The listing builds one solid part. Answer for the finished solid, in the listing's coordinates (mm). Face numbers are marked on the shaded views. A direction names the side the tool comes from. Give positions to 0.01 mm unless a question says otherwise; leave off trailing zeros. Order: outer loops, then holes, each group sorted by start corner. A loop starts at its lowest first (then second) coordinate and runs counter-clockwise, first axis right, second up.
```python
from build123d import *

# Parameters (mm, degrees)
SKETCH1_W           = 18
SKETCH1_H           = 30
BOSS_EXTRUDE1_DEPTH = 5
SKETCH2_W           = 30
SKETCH2_H           = 30
BOSS_EXTRUDE2_DEPTH = 5
SKETCH3_R           = 1.2
CUT_EXTRUDE1_DEPTH  = 5
FILLET1_R           = 6
BOSS_EXTRUDE3_START = 4
SKETCH4_R           = 3
SKETCH4_R_2         = 1.2
BOSS_EXTRUDE3_DEPTH = 4
SKETCH5_R           = 1.7
CUT_EXTRUDE2_DEPTH  = 24
SKETCH6_R           = 3
CUT_EXTRUDE3_DEPTH  = 24
FILLET2_R           = 3


with BuildPart() as part:
    # Sketch1 → Boss-Extrude1 (new body)
    with BuildSketch(Plane(origin=(0, 0, 0), x_dir=(1, 0, 0), z_dir=(0, 1, 0))):
        with Locations((9, 15)):
            Rectangle(SKETCH1_W, SKETCH1_H)
    extrude(amount=BOSS_EXTRUDE1_DEPTH)

    # Sketch2 → Boss-Extrude2 (add)
    with BuildSketch(Plane(origin=(18, 0, 0), x_dir=(0, 0, -1), z_dir=(1, 0, 0))):
        with Locations((15, 15)):
            Rectangle(SKETCH2_W, SKETCH2_H)
    extrude(amount=-BOSS_EXTRUDE2_DEPTH)

    # Sketch3 → Cut-Extrude1 (cut)
    with BuildSketch(Plane(origin=(18, 0, 0), x_dir=(0, 0, -1), z_dir=(1, 0, 0))):
        with Locations((4.25, 27)):
            Circle(SKETCH3_R)
        with Locations((25.75, 27)):
            Circle(SKETCH3_R)
        with Locations(Location((25.75, 14.5, 0), (0, 0, 180))):
            Circle(SKETCH3_R)
        with Locations(Location((4.25, 14.5, 0), (0, 0, 180))):
            Circle(SKETCH3_R)
    extrude(amount=-CUT_EXTRUDE1_DEPTH, mode=Mode.SUBTRACT)

    # Fillet1
    fillet1_edges = [part.edges().sort_by_distance(p)[0] for p in [
        (13, 5, -15),
        (18, 0, -15),
    ]]
    fillet(fillet1_edges, radius=FILLET1_R)

    # Sketch4 → Boss-Extrude3 (add)
    # profile 1 of 4: a face of its own
    with BuildSketch(Plane(origin=(18, 0, 0), x_dir=(0, 0, -1), z_dir=(1, 0, 0)).offset(BOSS_EXTRUDE3_START)):
        with Locations(Location((4.25, 27, 0), (0, 0, 90))):
            Circle(SKETCH4_R)
        with Locations((4.25, 27)):
            Circle(SKETCH4_R_2, mode=Mode.SUBTRACT)
    # profile 2 of 4: a face of its own
    with BuildSketch(Plane(origin=(18, 0, 0), x_dir=(0, 0, -1), z_dir=(1, 0, 0)).offset(BOSS_EXTRUDE3_START)):
        with Locations(Location((25.75, 27, 0), (0, 0, 90))):
            Circle(SKETCH4_R)
        with Locations((25.75, 27)):
            Circle(SKETCH4_R_2, mode=Mode.SUBTRACT)
    # profile 3 of 4: a face of its own
    with BuildSketch(Plane(origin=(18, 0, 0), x_dir=(0, 0, -1), z_dir=(1, 0, 0)).offset(BOSS_EXTRUDE3_START)):
        with Locations(Location((4.25, 14.5, 0), (0, 0, 180))):
            Circle(SKETCH4_R)
        with Locations((4.25, 14.5)):
            Circle(SKETCH4_R_2, mode=Mode.SUBTRACT)
    # profile 4 of 4: a face of its own
    with BuildSketch(Plane(origin=(18, 0, 0), x_dir=(0, 0, -1), z_dir=(1, 0, 0)).offset(BOSS_EXTRUDE3_START)):
        with Locations(Location((25.75, 14.5, 0), (0, 0, 180))):
            Circle(SKETCH4_R)
        with Locations((25.75, 14.5)):
            Circle(SKETCH4_R_2, mode=Mode.SUBTRACT)
    extrude(amount=-BOSS_EXTRUDE3_DEPTH)

    # Sketch5 → Cut-Extrude2 (cut)
    with BuildSketch(Plane.XZ):
        with Locations(Location((8, -5.510071499, 0), (0, 0, 270))):
            Circle(SKETCH5_R)
        with Locations(Location((8, -25.510071499, 0), (0, 0, 270))):
            Circle(SKETCH5_R)
    extrude(amount=-CUT_EXTRUDE2_DEPTH, mode=Mode.SUBTRACT)

    # Sketch6 → Cut-Extrude3 (cut)
    with BuildSketch(Plane(origin=(0, 5, 0), x_dir=(1, 0, 0), z_dir=(0, 1, 0))):
        with Locations((8, 25.510071499)):
            Circle(SKETCH6_R)
        with Locations((8, 5.510071499)):
            Circle(SKETCH6_R)
    extrude(amount=CUT_EXTRUDE3_DEPTH, mode=Mode.SUBTRACT)

    # Fillet2
    fillet2_edges = [part.edges().sort_by_distance(p)[0] for p in [
        (0, 2.5, -30),
        (0, 2.5, 0),
    ]]
    fillet(fillet2_edges, radius=FILLET2_R)


solid = part.part
```
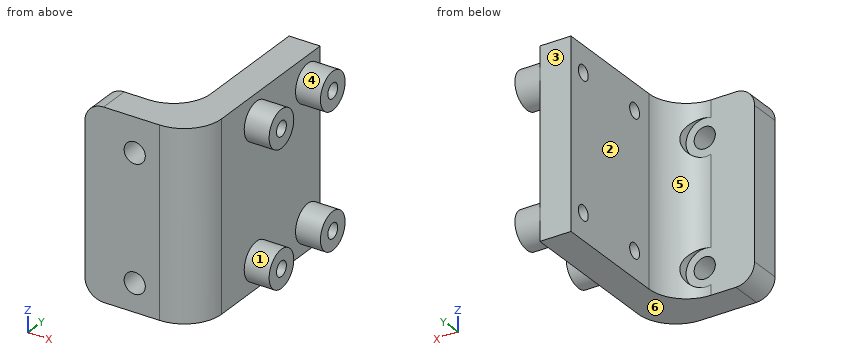
1) Find section A-A (y = 27). Write down the section's boundary in (x, z).
Geometry says:
outline: (13, -30) - (18, -30) - (18, -28.75) - (22, -28.75) - (22, -26.95) - (13, -26.95) - close; (13, -24.55) - (22, -24.55) - (22, -22.75) - (18, -22.75) - (18, -7.25) - (22, -7.25) - (22, -5.45) - (13, -5.45) - close; (13, -3.05) - (22, -3.05) - (22, -1.25) - (18, -1.25) - (18, 0) - (13, 0) - close
2) A tool of negligible diameter and unlimited length cuts with its end or side. For the marked faces 1, 2 and 3, from which of +Z, -Z, +X, -X, +Y, -Y can it reach the whole face along a straight path? Write none if from no direction.
Geometry says:
face 1: +X
face 2: +Z, -Z, -X, +Y
face 3: +Z, -Z, +X, -X, +Y
3) Find section D-D (y = 20). Write down the section's boundary in (x, z).
Geometry says:
outline: (13, -30) - (18, -30) - (18, 0) - (13, 0) - close
4) Find section C-C (x = 17.5). Write down the section's boundary in (y, z).
Geometry says:
outline: (3.6, -30) - (30, -30) - (30, 0) - (3.6, 0) - close; hole circle Ø2.4 at (14.5, -25.75); hole circle Ø2.4 at (14.5, -4.25); hole circle Ø2.4 at (27, -25.75); hole circle Ø2.4 at (27, -4.25)
5) Find section B-B (x = 8). Write down the section's boundary in (y, z), then the cut area to 3 significant figures.
Geometry says:
outline: (0, -30) - (5.08, -30) - (5.08, -28.51) - (5, -28.51) - (5, -27.21) - (0, -27.21) - close; (0, -23.81) - (5, -23.81) - (5, -22.51) - (5.08, -22.51) - (5.08, -8.51) - (5, -8.51) - (5, -7.21) - (0, -7.21) - close; (0, -3.81) - (5, -3.81) - (5, -2.51) - (5.08, -2.51) - (5.08, 0) - (0, 0) - close
area: 118 mm2
6) Straight lines are drawn through the part: probe 1 along Z at (x, y) = (20.5, 27.5); probe 2 along Y at (x, z) = (17, -4.25); probe 3 along Y at (x, z) = (5.5, -12.5). For each, find the intervals that lie inside material, in ascending order.
Geometry says:
probe 1: z = -28.71 to -26.84, -24.66 to -22.79, -7.21 to -5.34, -3.16 to -1.29
probe 2: y = 2.68 to 13.3, 15.7 to 25.8, 28.2 to 30
probe 3: y = 0 to 5
7) For a pull along Y with two mould halves and no side action, classify the marked faces 4, 5 and 6 as +Y half, -Y half, draft (parallel to the pull), parting line (faces both ways), or undercut.
Geometry says:
face 4: undercut
face 5: +Y half
face 6: draft
8) Given P1, Ø4, axis at y = 14.5, z = -25.75, coming from the -X side; P2, Ø9, axis at x = 4, z = -12, coming from the +Y side, each flat-ended and moving along its own axis, determine where each tip first touches the part or whether it passes through.
Geometry says:
P1: stops at x = 13
P2: stops at y = 5.19
